```python
from build123d import *

# Parameters (mm, degrees)
BOSS_EXTRUDE1_DEPTH = 50
BOSS_EXTRUDE3_DEPTH = 29.899298
SKETCH3_R           = 3
CUT_EXTRUDE1_DEPTH  = 30.899298
SKETCH4_R           = 3
CUT_EXTRUDE2_DEPTH  = 38.007847
FILLET1_R           = 3
CHAMFER1_SIZE       = 1


with BuildPart() as part:
    # Sketch1 → Boss-Extrude1 (new body)
    with BuildSketch(Plane.XY):
        Polygon((0, 15), (14.899298, 15), (14.899298, -14.949649), (-15, -14.949649), (-15, 15), align=None)
        Polygon((-9.966433, 9.966433), (-4.741433, 9.966433), (-3.1, 8.307461), (-5.5, 8.307461), (-5.5, 6.667461), (-2.79, 3.957461), (2.79, 3.957461), (5.5, 6.667461), (5.5, 8.307461), (3.1, 8.307461), (4.741433, 9.966433), (9.966433, 9.966433), (9.966433, 4.741433), (8.307461, 3.1), (8.307461, 5.5), (6.667461, 5.5), (3.957461, 2.79), (3.957461, -2.79), (6.667461, -5.5), (8.307461, -5.5), (8.307461, -3.1), (9.966433, -4.741433), (9.966433, -9.966433), (4.741433, -9.966433), (3.1, -8.307461), (5.5, -8.307461), (5.5, -6.667461), (2.79, -3.957461), (-2.79, -3.957461), (-5.5, -6.667461), (-5.5, -8.307461), (-3.1, -8.307461), (-4.741433, -9.966433), (-9.966433, -9.966433), (-9.966433, -4.741433), (-8.307461, -3.1), (-8.307461, -5.5), (-6.667461, -5.5), (-3.957461, -2.79), (-3.957461, 2.79), (-6.667461, 5.5), (-8.307461, 5.5), (-8.307461, 3.1), (-9.966433, 4.741433), align=None, mode=Mode.SUBTRACT)
    extrude(amount=BOSS_EXTRUDE1_DEPTH)

    # Sketch5 → Boss-Extrude3 (add, through all)
    with BuildSketch(Plane.ZY.offset(15)):
        with BuildLine():
            Line((0, 26), (0, 15))
            Line((0, 15), (17, 15))
            ThreePointArc((17, 15), (13.683375, 36.488088), (23.324555, 17))
            Line((23.324555, 17), (27.804488, 17))
            Line((27.804488, 17), (50, 17))
            Line((50, 17), (50, 21))
            Line((50, 21), (33.248077, 21))
            ThreePointArc((33.248077, 21), (19.528111, 42.810968), (0, 26))
        make_face()
    extrude(amount=-BOSS_EXTRUDE3_DEPTH)

    # Sketch3 → Cut-Extrude1 (cut, through all)
    with BuildSketch(Plane.ZY.offset(15)):
        with Locations((12, 0)):
            Circle(SKETCH3_R)
        with Locations((27, 0)):
            Circle(SKETCH3_R)
    extrude(amount=-CUT_EXTRUDE1_DEPTH, mode=Mode.SUBTRACT)

    # Sketch4 → Cut-Extrude2 (cut, through all)
    with BuildSketch(Plane(origin=(0, 22.058198, 0), x_dir=(1, 0, 0), z_dir=(0, 1, 0))):
        with Locations((0, -42.5)):
            Circle(SKETCH4_R)
    extrude(amount=-CUT_EXTRUDE2_DEPTH, mode=Mode.SUBTRACT)

    # Fillet1
    fillet1_edges = [part.edges().sort_by_distance(p)[0] for p in [
        (-0.050351, -14.949649, 50),
        (14.899298, 0.025175, 50),
        (14.899298, 42.810968, 19.528111),
        (14.899298, 21, 41.624038),
        (14.899298, 19, 50),
        (-0.050351, 21, 50),
        (-15, 19, 50),
        (-15, 21, 41.624038),
        (-15, 42.810968, 19.528111),
        (14.899298, 0.025175, 0),
        (-0.050351, -14.949649, 0),
        (-15, 5.525175, 0),
        (-15, 0.025175, 50),
        (14.899298, -14.949649, 25),
        (-15, -14.949649, 25),
    ]]
    fillet(fillet1_edges, radius=FILLET1_R)

    # Chamfer1
    chamfer1_edges = [part.edges().sort_by_distance(p)[0] for p in [
        (14.899298, 0, 9),
        (-15, 0, 9),
        (14.899298, 0, 24),
        (-15, 0, 24),
        (-3, -14.949649, 42.5),
        (-3, 21, 42.5),
    ]]
    chamfer(chamfer1_edges, length=CHAMFER1_SIZE)


solid = part.part
```
Work out the finished part from the listing and answer in its coordinate system (mm). A direction names the side the tool comes from. Coordinates: 2 decimals unless noted, no trailing zeros. Order: outer loops, then holes, each group sorted by start corner. A loop starts at its lowest first (then second) coordinate and runs counter-clockwise, first axis right, second up. Notation, with made-up numbers: (-21, 37) - (10, 37) arc R27 cw to (10, 53) - close; hole circle Ø7 at (74.5, 11.5). An arc over 180 degrees is marked (long way). Answer as a JSON object with one key per item and string values.
1. Find section B-B on y = 14. Determine the outline of the cut face in (x, z), plus the area to 3 significant figures.
Output values:
{"outline": "(-15, 3) arc R3 ccw to (-12, 0) - (11.9, 0) arc R3 ccw to (14.9, 3) - (14.9, 47) arc R3 ccw to (11.9, 50) - (-12, 50) arc R3 ccw to (-15, 47) - close; hole circle Ø6 at (0, 42.5)", "area": "1,460 mm²"}
2. Consider line 1 (X direction, y = -8, z = 36); line 2 (Z direction, x = -8, y = 0); line 3 (X direction, y = 18.2, z = 42.5). Determine where each line is inside the solid, lowest interval first.
Output values:
{"line 1": "x = -15 to -9.97, -5.5 to 5.5, 9.97 to 14.9", "line 2": "z = 0 to 9, 15 to 24, 30 to 50", "line 3": "x = -14.99 to -3, 3 to 14.89"}
3. A tool of negligible diameter and unlimited length cuts with its end or side. For faces 4 (the face through (-0.26, 36.35, 13.27)), 5 (the face through (3.957, 0, 19)), from which of +Z, -Z, +X, -X, +Y, -Y can it reach the whole face along a straight path? Write none if from no direction.
Output values:
{"face 4": "+X, -X", "face 5": "+Z, -Z"}
4. Each of these flat-tipped pins is pushed along its axis until it touches: P1, Ø5, axis at x = 3, y = 30.5, coming from the +Z side; P2, Ø4, axis at x = 4.5, z = 21, coming from the +Y side; P3, Ø6, axis at x = 0.5, y = 36, coming from the +Z side. Where does it stop, or does it pass through?
Output values:
{"P1": "stops at z = 33.88", "P2": "stops at y = 42.88", "P3": "stops at z = 32.49"}
5. The mould has two halves that part along Y. Classify faces 1 (the face through (7, 5.5, 25)), 2 (the face through (5.5, 7, 25)), 3 (the face through (14.04, 17.51, 49.1)): +Y half, -Y half, draft (parallel to the pull), parting line (faces both ways), or undercut.
Output values:
{"face 1": "undercut", "face 2": "undercut", "face 3": "draft"}
6. Find section A-A on x = 0. Count the separate pieces of the cut face and the enclosed holes in it, plus the area to 3 significant figures.
Output values:
{"separate pieces": "5", "enclosed holes": "0", "area": "1,420 mm²"}
